from build123d import *

# Parameters (mm, degrees)
F0_R     = 9.525
F1_DEPTH = 25.4
F2_R     = 6.35
F3_DEPTH = 7.9375
F4_R     = 3.96875
F5_DEPTH = 17.4635


with BuildPart() as f1:
    # F0 (on Right) → F1 (new body)
    with BuildSketch(Plane.YZ):
        Circle(F0_R)
    extrude(amount=F1_DEPTH)

    # F2 (on face) → F3 (cut)
    with BuildSketch(Plane.YZ.offset(25.4)):
        Circle(F2_R)
    extrude(amount=-F3_DEPTH, mode=Mode.SUBTRACT)

    # F4 (on face) → F5 (cut, through all)
    with BuildSketch(Plane.YZ.offset(17.4625)):
        Circle(F4_R)
    extrude(amount=-F5_DEPTH, mode=Mode.SUBTRACT)


solid = f1.part
For this review, take the finished solid that the model builds, in its own axes (mm). A direction names the side the tool comes from. Coordinates: 2 decimals unless noted, no trailing zeros. Order: outer loops, then holes, each group sorted by start corner. A loop starts at its lowest first (then second) coordinate and runs counter-clockwise, first axis right, second up. Notation, with made-up numbers: (25.5, 51.25) - (45.5, 51.25) arc R30 cw to (45.5, 80.25) - close; hole circle Ø8 at (14, 84.5). An arc over 180 degrees is marked (long way). Use one line per item in the form item = value.
Q1. For P1, Ø4, axis at y = 0.5, z = -1, coming from the +X side; P2, Ø8, axis at x = 20.5, z = -7, coming from the +Y side, all flat-tipped, find the tip position at first contact; note any pin that passes through.
Checked values:
P1 = through
P2 = 9.04
Q2. Consider section B-B (z = -2.5). Give the boundary of the cut face in (x, y), then the cut area to 3 significant figures.
Checked values:
outline = (0, -9.19) - (25.4, -9.19) - (25.4, -5.84) - (17.46, -5.84) - (17.46, -3.08) - (0, -3.08) - close; (0, 3.08) - (17.46, 3.08) - (17.46, 5.84) - (25.4, 5.84) - (25.4, 9.19) - (0, 9.19) - close
area = 267 mm2
Q3. For probe 1 along Z at (x, y) = (7.75, 0) (3 decimals); probe 2 along Z at (x, y) = (20.5, 0) (3 decimals); probe 3 along Y at (x, z) = (2.5, 1), list the stretches that pass through material, from the lowest coordinate up. Write a range as from..to.
Checked values:
probe_1 = -9.525..-3.969, 3.969..9.525
probe_2 = -9.525..-6.35, 6.35..9.525
probe_3 = -9.47..-3.84, 3.84..9.47
Q4. For faces 4 (the cylindrical face through (8.853, -0.86, -3.874)), 5 (the flat face through (17.462, 3, 3)), list the 3-axis set-ups (+Z, -Z, +X, -X, +Y, -Y) from which the entire face can be reached by the end or side of a thin tool; tool diameter is ignored.
Checked values:
face_4 = +X, -X
face_5 = +X
Q5. Consider section D-D (y = -5.5). Give the boundary of the cut face in (x, z).
Checked values:
outline = (0, -7.78) - (25.4, -7.78) - (25.4, -3.17) - (17.46, -3.17) - (17.46, 3.17) - (25.4, 3.17) - (25.4, 7.78) - (0, 7.78) - close
Q6. Draft analysis for pull direction Z (two halves, no side actions). For faces 1 (the cylindrical face through (12.522, -7.559, -5.796)), 2 (the flat face through (25.4, 2, -6.2)), 3 (the cylindrical face through (21.49, -1.38, -6.2)), state which applies: +Z half, -Z half, draft (parallel to the pull), parting line (faces both ways), or undercut.
Checked values:
face_1 = parting line
face_2 = draft
face_3 = undercut
